from build123d import *

# Parameters (mm, degrees)
SKETCH2_R           = 2.499990149
BOSS_EXTRUDE1_DEPTH = 10
FILLET1_R           = 1


with BuildPart() as part:
    # Sketch2 → Boss-Extrude1 (new body)
    with BuildSketch(Plane.XY):
        Polygon((0, 0), (0, 90), (55, 90), (55, 65), (20, 65), (20, 0), align=None)
        with Locations((42.025587792, 80.329294261)):
            Circle(SKETCH2_R, mode=Mode.SUBTRACT)
    extrude(amount=BOSS_EXTRUDE1_DEPTH)

    # Fillet1
    fillet1_edges = [part.edges().sort_by_distance(p)[0] for p in [
        (0, 0, 5),
        (0, 90, 5),
        (55, 90, 5),
        (55, 65, 5),
        (20, 65, 5),
        (20, 0, 5),
        (37.5, 65, 10),
        (55, 77.5, 10),
        (27.5, 90, 10),
        (0, 45, 10),
        (10, 0, 10),
        (0, 45, 0),
        (27.5, 90, 0),
        (55, 77.5, 0),
        (37.5, 65, 0),
        (20, 32.5, 0),
        (10, 0, 0),
        (20, 32.5, 10),
    ]]
    fillet(fillet1_edges, radius=FILLET1_R)


solid = part.part
Source: CAD feature listing. Evaluate the final solid. Frame: model axes, mm. Round coordinates to 2 decimals unless told otherwise and drop trailing zeros. Loops run counter-clockwise (first coordinate to the right, second up) from the corner with the lowest first, then second, coordinate; pieces in that order, holes last.
Q1. First-contact query: P1, Ø5, axis at y = 31, z = 8, coming from the +X side; P2, Ø6, axis at x = 29.5, z = 2, coming from the -Y side. Flat tips, straight axial feed; report the tip coordinate or a pass-through.
Q2. Section A-A, the plane y = 56. Return loops of the section in (x, z).
Q3. Section C-C, the plane z = 5.5. Return loops of the section in (x, y), plus the area to 3 significant figures.
Q4. Section D-D, the plane x = 35.5. Return loops of the section in (y, z), plus the area to 3 significant figures.
Q5. Section B-B, the plane x = 43.5. Return loops of the section in (y, z).
Q6. Mould query, pull axis Y, two halves, no side actions, for faces 1 (the face through (44.335, 79.372, 4.93)), 2 (the face through (38, 65, 5)), 3 (the face through (20, 33, 5)). Classes: pulls with the +Y half, pulls with the -Y half, needs draft (parallel to the pull), parting line crosses it, or undercut.
Q7. Ray query, line 1 (X direction, y = 29.5, z = 1.25); line 2 (Y direction, x = 49.5, z = 7.5); line 3 (X direction, y = 82.5, z = 9.25). Return the intervals inside material, ascending.
Solutions:
1. P1: stops at x = 20
1. P2: stops at y = 65
2. outline: (0, 1) arc R1 ccw to (1, 0) - (19, 0) arc R1 ccw to (20, 1) - (20, 9) arc R1 ccw to (19, 10) - (1, 10) arc R1 ccw to (0, 9) - close
3. outline: (0, 1) arc R1 ccw to (1, 0) - (19, 0) arc R1 ccw to (20, 1) - (20, 64) arc R1 cw to (21, 65) - (54, 65) arc R1 ccw to (55, 66) - (55, 89) arc R1 ccw to (54, 90) - (1, 90) arc R1 ccw to (0, 89) - close; hole circle Ø5 at (42.03, 80.33)
3. area: 2,650 mm2
4. outline: (65, 1) arc R1 ccw to (66, 0) - (89, 0) arc R1 ccw to (90, 1) - (90, 9) arc R1 ccw to (89, 10) - (66, 10) arc R1 ccw to (65, 9) - close
4. area: 249 mm2
5. outline: (65, 1) arc R1 ccw to (66, 0) - (78.31, 0) - (78.31, 10) - (66, 10) arc R1 ccw to (65, 9) - close; (82.35, 0) - (89, 0) arc R1 ccw to (90, 1) - (90, 9) arc R1 ccw to (89, 10) - (82.35, 10) - close
6. face 1: undercut
6. face 2: pulls with the -Y half
6. face 3: needs draft
7. line 1: x = 0 to 20
7. line 2: y = 65 to 90
7. line 3: x = 0.03 to 40.79, 43.27 to 54.97
